from build123d import *

# Parameters (mm, degrees)
SKETCH001_R       = 0.6
PAD001_DEPTH      = 12
PAD001_DEPTH_BACK = 3.5
SKETCH_R          = 12
PAD_DEPTH         = 24
FILLET_R          = 0.5


with BuildPart() as pad001:
    # Sketch001 → Pad001 (new body, two sides)
    with BuildSketch(Plane.XY.offset(0.5)) as pad001_sk:
        Circle(SKETCH001_R)
        with Locations((24, 0)):
            Circle(SKETCH001_R)
    extrude(amount=PAD001_DEPTH)
    extrude(pad001_sk.sketch, amount=-PAD001_DEPTH_BACK)


with BuildPart() as l_radial_d24_0mm_p24_00mm:
    # Sketch → Pad (new body)
    with BuildSketch(Plane.XY.offset(0.1)):
        with Locations((12, 0)):
            Circle(SKETCH_R)
    extrude(amount=PAD_DEPTH)

    # Fillet
    fillet_edges = [l_radial_d24_0mm_p24_00mm.edges().sort_by_distance(p)[0] for p in [
        (0, 0, 0.1),
        (0, 0, 24.1),
    ]]
    fillet(fillet_edges, radius=FILLET_R)

    add(pad001.part)


solid = l_radial_d24_0mm_p24_00mm.part
CAD build for the part. Positions are in the model's coordinates, mm. A direction names the side the tool comes from. Round coordinates to 2 decimals unless told otherwise and drop trailing zeros. Write each loop counter-clockwise with the first axis right and the second up, starting at its lowest first coordinate (ties: lowest second). Pieces come first, ordered by that corner, then holes. Notation, with made-up numbers: (53.5, -12.75) -> (70.5, -12.75) arc R21 cw to (70.5, 21.25) -> close; hole circle Ø11 at (-22.75, 15.5). An arc over 180 degrees is marked (long way). Answer as a JSON object with one key per item and string values.
(1) Band-saw the part on C-C, the plane z = 10.5. List the corners of the cut face in (x, y) (3 decimals).
Reported:
{"outline": "(0.015, -0.6) arc R12 ccw to (23.985, -0.6) arc R0.6 ccw (long way) to (23.985, 0.6) arc R12 ccw to (0.015, 0.6) arc R0.6 ccw (long way) to start"}
(2) Which spindle directions (+Z, -Z, +X, -X, +Y, -Y) get a long thin tool onto all of the face, cutting with end or side? Do faces 1 (the face through (12, 0, 24.1)), 2 (the face through (24.554, -0.23, 3.136)). Say none if no direction does.
Reported:
{"face 1": "+Z, +X, -X, +Y, -Y", "face 2": "-Z"}
(3) Band-saw the part on B-B, the plane z = 14.25. List the corners of the cut face in (x, y), then the cut area to 3 significant figures.
Reported:
{"outline": "circle Ø24 at (12, 0)", "area": "452 mm^2"}
(4) Pin check, flat tips, straight feed: P1, Ø3, axis at x = 17.5, y = -4, coming from the -Z side; P2, Ø1.5, axis at x = 15, z = 6, coming from the +Y side; P3, Ø2, axis at y = 9.5, z = 15, coming from the -X side. Stop position of each tip, or through.
Reported:
{"P1": "stops at z = 0.1", "P2": "stops at y = 11.79", "P3": "stops at x = 3.53"}
(5) Band-saw the part on A-A, the plane x = 12. List the corners of the cut face in (y, z), then the cut area to 3 significant figures.
Reported:
{"outline": "(-12, 0.6) arc R0.5 ccw to (-11.5, 0.1) -> (11.5, 0.1) arc R0.5 ccw to (12, 0.6) -> (12, 23.6) arc R0.5 ccw to (11.5, 24.1) -> (-11.5, 24.1) arc R0.5 ccw to (-12, 23.6) -> close", "area": "576 mm^2"}
(6) Probe probe 1 along Z at (x, y) = (12.25, 11.25); probe 2 along X at (y, z) = (3.75, 3); probe 3 along X at (y, z) = (-5, 19). List the from-to ranges inside material, lowest first. Write a range as [from, to].
Reported:
{"probe 1": "z = [0.1, 24.1]", "probe 2": "x = [0.6, 23.4]", "probe 3": "x = [1.09, 22.91]"}
